Input: part model. Units: mm. Frame: model coordinates. Face numbers are marked on the shaded views. Round coordinates to 2 decimals unless told otherwise and drop trailing zeros. Order: outer loops, then holes, each group sorted by start corner. A loop starts at its lowest first (then second) coordinate and runs counter-clockwise, first axis right, second up. Notation, with made-up numbers: (72, 8.25) - (94, 8.25) arc R23 ccw to (94, 41.25) - close; hole circle Ø2 at (51, 85.5). An arc over 180 degrees is marked (long way). One line per item, written item: value. Start each with the question number.
from build123d import *

# Parameters (mm, degrees)
SKETCH007_W     = 116.5
SKETCH007_H     = 84
PAD002_DEPTH    = 2
SKETCH008_W     = 112.5
SKETCH008_H     = 80
PAD003_DEPTH    = 2
SKETCH009_W     = 108.5
SKETCH009_H     = 76
POCKET004_DEPTH = 2
FILLET008_R     = 1
SKETCH010_W     = 2
SKETCH010_H     = 8
PAD004_DEPTH    = 8
FILLET010_R     = 3
SKETCH011_R     = 1.25
POCKET005_DEPTH = 2
SKETCH012_W     = 2
SKETCH012_H     = 8
PAD005_DEPTH    = 8
SKETCH013_W     = 2
SKETCH013_H     = 8
PAD006_DEPTH    = 8
SKETCH014_W     = 2
SKETCH014_H     = 8
PAD007_DEPTH    = 8
FILLET011_R     = 3
FILLET012_R     = 3
FILLET013_R     = 3
SKETCH015_R     = 1.25
POCKET006_DEPTH = 5
SKETCH016_R     = 1.25
POCKET007_DEPTH = 5
SKETCH017_R     = 1.25
POCKET008_DEPTH = 5
FILLET014_R     = 1
FILLET015_R     = 1
FILLET016_R     = 1
SKETCH018_W     = 88.5656
SKETCH018_H     = 13.4224
POCKET009_DEPTH = 0.2
SKETCH019_W     = 85.956
SKETCH019_H     = 9.716
POCKET010_DEPTH = 0.2
CHAMFER006_SIZE = 0.2
CHAMFER007_SIZE = 0.2
CHAMFER008_SIZE = 0.2
CHAMFER009_SIZE = 0.2


with BuildPart() as part:
    # Sketch007 → Pad002 (new body)
    with BuildSketch(Plane(origin=(0, 0, 0), x_dir=(1, 0, 0), z_dir=(0, 0, -1))):
        with Locations((58.25, 42)):
            Rectangle(SKETCH007_W, SKETCH007_H)
    extrude(amount=PAD002_DEPTH)

    # Sketch008 (on Face5 of Pad002) → Pad003 (new body)
    with BuildSketch(Plane.XY):
        with Locations((58.25, -42)):
            Rectangle(SKETCH008_W, SKETCH008_H)
    extrude(amount=PAD003_DEPTH)

    # Sketch009 (on Face11 of Pad003) → Pocket004 (cut)
    with BuildSketch(Plane.XY.offset(2)):
        with Locations((58.25, -42)):
            Rectangle(SKETCH009_W, SKETCH009_H)
    extrude(amount=-POCKET004_DEPTH, mode=Mode.SUBTRACT)

    # Fillet008
    fillet008_edges = [part.edges().sort_by_distance(p)[0] for p in [
        (0, 0, -1),
        (116.5, 0, -1),
        (0, -84, -1),
        (116.5, -84, -1),
        (114.5, -82, 1),
        (2, -82, 1),
        (114.5, -2, 1),
        (2, -2, 1),
    ]]
    fillet(fillet008_edges, radius=FILLET008_R)

    # Sketch010 (on Face19 of Fillet008) → Pad004 (new body)
    with BuildSketch(Plane.XY.offset(2)):
        with Locations((3, -8)):
            Rectangle(SKETCH010_W, SKETCH010_H)
    extrude(amount=PAD004_DEPTH)

    # Fillet010
    fillet010_edges = [part.edges().sort_by_distance(p)[0] for p in [
        (3, -4, 10),
        (3, -12, 10),
    ]]
    fillet(fillet010_edges, radius=FILLET010_R)

    # Sketch011 (on Face5 of Fillet010) → Pocket005 (cut)
    with BuildSketch(Plane(origin=(2, 0, 0), x_dir=(0, -1, 0), z_dir=(-1, 0, 0))):
        with Locations((8, 6)):
            Circle(SKETCH011_R)
    extrude(amount=-POCKET005_DEPTH, mode=Mode.SUBTRACT)

    # Sketch012 (on Face11 of Pocket005) → Pad005 (new body)
    with BuildSketch(Plane.XY.offset(2)):
        with Locations((3, -76)):
            Rectangle(SKETCH012_W, SKETCH012_H)
    extrude(amount=PAD005_DEPTH)

    # Sketch013 (on Face11 of Pad005) → Pad006 (new body)
    with BuildSketch(Plane.XY.offset(2)):
        with Locations((113.5, -8)):
            Rectangle(SKETCH013_W, SKETCH013_H)
    extrude(amount=PAD006_DEPTH)

    # Sketch014 (on Face20 of Pad006) → Pad007 (new body)
    with BuildSketch(Plane.XY.offset(2)):
        with Locations((113.5, -76)):
            Rectangle(SKETCH014_W, SKETCH014_H)
    extrude(amount=PAD007_DEPTH)

    # Fillet011
    fillet011_edges = [part.edges().sort_by_distance(p)[0] for p in [
        (113.5, -72, 10),
        (113.5, -80, 10),
    ]]
    fillet(fillet011_edges, radius=FILLET011_R)

    # Fillet012
    fillet012_edges = [part.edges().sort_by_distance(p)[0] for p in [
        (113.5, -4, 10),
        (113.5, -12, 10),
    ]]
    fillet(fillet012_edges, radius=FILLET012_R)

    # Fillet013
    fillet013_edges = [part.edges().sort_by_distance(p)[0] for p in [
        (3, -72, 10),
        (3, -80, 10),
    ]]
    fillet(fillet013_edges, radius=FILLET013_R)

    # Sketch015 (on Face2 of Fillet013) → Pocket006 (cut)
    with BuildSketch(Plane(origin=(2, 0, 0), x_dir=(0, -1, 0), z_dir=(-1, 0, 0))):
        with Locations((76, 6)):
            Circle(SKETCH015_R)
    extrude(amount=-POCKET006_DEPTH, mode=Mode.SUBTRACT)

    # Sketch016 (on Face25 of Pocket006) → Pocket007 (cut)
    with BuildSketch(Plane.YZ.offset(114.5)):
        with Locations((-76, 6)):
            Circle(SKETCH016_R)
    extrude(amount=-POCKET007_DEPTH, mode=Mode.SUBTRACT)

    # Sketch017 (on Face24 of Pocket007) → Pocket008 (cut)
    with BuildSketch(Plane.YZ.offset(114.5)):
        with Locations((-8, 6)):
            Circle(SKETCH017_R)
    extrude(amount=-POCKET008_DEPTH, mode=Mode.SUBTRACT)

    # Fillet014
    fillet014_edges = [part.edges().sort_by_distance(p)[0] for p in [
        (113.5, -72, 2),
    ]]
    fillet(fillet014_edges, radius=FILLET014_R)

    # Fillet015
    fillet015_edges = [part.edges().sort_by_distance(p)[0] for p in [
        (3, -72, 2),
        (3, -12, 2),
    ]]
    fillet(fillet015_edges, radius=FILLET015_R)

    # Fillet016
    fillet016_edges = [part.edges().sort_by_distance(p)[0] for p in [
        (113.5, -12, 2),
    ]]
    fillet(fillet016_edges, radius=FILLET016_R)

    # Sketch018 (on Face46 of Fillet016) → Pocket009 (cut)
    with BuildSketch(Plane(origin=(2, 0, 0), x_dir=(0, -1, 0), z_dir=(-1, 0, 0))):
        with Locations((42.9281, 8.7112)):
            Rectangle(SKETCH018_W, SKETCH018_H)
    extrude(amount=-POCKET009_DEPTH, mode=Mode.SUBTRACT)

    # Sketch019 (on Face4 of Pocket009) → Pocket010 (cut)
    with BuildSketch(Plane.YZ.offset(114.5)):
        with Locations((-38.022, 6.858)):
            Rectangle(SKETCH019_W, SKETCH019_H)
    extrude(amount=-POCKET010_DEPTH, mode=Mode.SUBTRACT)

    # Chamfer006
    chamfer006_edges = [part.edges().sort_by_distance(p)[0] for p in [
        (114.3, -9.25, 6),
    ]]
    chamfer(chamfer006_edges, length=CHAMFER006_SIZE)

    # Chamfer007
    chamfer007_edges = [part.edges().sort_by_distance(p)[0] for p in [
        (114.3, -77.25, 6),
    ]]
    chamfer(chamfer007_edges, length=CHAMFER007_SIZE)

    # Chamfer008
    chamfer008_edges = [part.edges().sort_by_distance(p)[0] for p in [
        (2.2, -74.75, 6),
        (2.2, -6.75, 6),
        (4, -6.75, 6),
        (4, -74.75, 6),
    ]]
    chamfer(chamfer008_edges, length=CHAMFER008_SIZE)

    # Chamfer009
    chamfer009_edges = [part.edges().sort_by_distance(p)[0] for p in [
        (112.5, -77.25, 6),
        (112.5, -9.25, 6),
    ]]
    chamfer(chamfer009_edges, length=CHAMFER009_SIZE)


solid = part.part
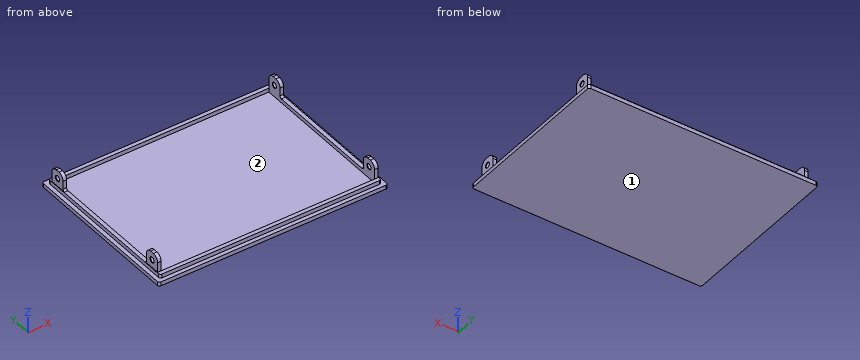
Item 1: Pull-direction query (Y, two-part tool) for the marked faces 1 and 2; classes: released by +Y, released by -Y, zero draft, split by the parting line, or undercut.
Item 2: First-contact query: pin 1 Ø6 at (y, z) = (-34.5, 4.5) entering from -X; pin 2 Ø1.4 at (x, z) = (113.5, 4.5) entering from +Y; pin 3 Ø0.9 at (x, z) = (3, 4) entering from -Y; pin 4 Ø2 at (x, z) = (47, 0.5) entering from +Y. Flat tips, straight axial feed; report the tip coordinate or a pass-through.
Item 3: Section query B-B on y = -25.5. Return loops of the section in (x, z), and give its area (3 significant figures).
Item 4: Section query A-A on x = 32.5. Return loops of the section in (y, z).
Item 5: Line query: L1, parallel to X at y = -26, z = 0.5; L2, parallel to Z at x = 113.3, y = -76; L3, parallel to Y at x = 99, z = 0.5. Output: solid intervals per line, ascending.
Geometry results:
1. face 1: zero draft
1. face 2: undercut
2. pin 1: stops at x = 2
2. pin 2: stops at y = -4
2. pin 3: stops at y = -80
2. pin 4: stops at y = 0
3. outline: (0, -2) - (116.5, -2) - (116.5, 0) - (114.5, 0) - (114.5, 2) - (112.5, 2) - (112.5, 0) - (4, 0) - (4, 2) - (2, 2) - (2, 0) - (0, 0) - close
3. area: 241 mm^2
4. outline: (-84, -2) - (0, -2) - (0, 0) - (-2, 0) - (-2, 2) - (-4, 2) - (-4, 0) - (-80, 0) - (-80, 2) - (-82, 2) - (-82, 0) - (-84, 0) - close
5. L1: x = 2 to 4, 112.5 to 114.5
5. L2: z = -2 to 4.75, 7.25 to 10
5. L3: y = -82 to -80, -4 to -2
